The model under review builds one solid part; all positions refer to its coordinate system, in mm. A direction names the side the tool comes from. Coordinates: 2 decimals unless noted, no trailing zeros. Write each loop counter-clockwise with the first axis right and the second up, starting at its lowest first coordinate (ties: lowest second). Pieces come first, ordered by that corner, then holes.
```python
from build123d import *

# Parameters (mm, degrees)
SKETCH3_W = 6
SKETCH3_H = 2.2


with BuildPart() as part:
    # Sweep1: sweep along a path in Sketch1
    with BuildLine(Plane(origin=(0, 0, 0), x_dir=(0, 0, -1), z_dir=(1, 0, 0))) as sweep1_path:
        Line((0.31090006, -5.3474047), (403.879965212, 18.116247973))
        ThreePointArc((403.879965212, 18.116247973), (415.790396806, 31.112194288), (403.14572952, 43.394921614))
        Line((403.14572952, 43.394921614), (20.942535542, 43.394921614))
        ThreePointArc((20.942535542, 43.394921614), (13.956361094, 41.290814966), (9.294242947, 35.678457834))
        Line((9.294242947, 35.678457834), (-4.932278427, 2.089024985))
        ThreePointArc((-4.932278427, 2.089024985), (-4.377716999, -3.086582212), (0.31090006, -5.3474047))
    # Sketch3 → Sweep1 (sweep)
    with BuildSketch(Plane(origin=(0, 2.089024985, 4.932278427), x_dir=(1, 0, 0), z_dir=(0, -0.920813644, 0.390002863))):
        with Locations((0, 1.1)):
            Rectangle(SKETCH3_W, SKETCH3_H)
    sweep(path=sweep1_path.line)


solid = part.part
```
Item 1: Take a section at C-C, the plane z = -76.5. Write out the cut boundary in (x, y).
Solved:
outline: (-3, -3.12) - (3, -3.12) - (3, -0.92) - (-3, -0.92) - close; (-3, 43.39) - (3, 43.39) - (3, 45.59) - (-3, 45.59) - close
Item 2: To check wall thickness, follow line 1 along Y through (x, z) = (1.7, -47.5); line 2 along Y through (x, z) = (-2.2, -370); line 3 along Z through (x, y) = (-0.25, 30). State the ranges of each line that lie inside material, in increasing order.
Solved:
line 1: y = -4.81 to -2.6, 43.39 to 45.59
line 2: y = 13.94 to 16.15, 43.39 to 45.59
line 3: z = -417.98 to -415.77, -6.89 to -4.5
Item 3: Take a section at A-A, the plane y = 29. Write out the cut boundary in (x, z), plus the area to 3 significant figures.
Solved:
outline: (-3, -417.89) - (3, -417.89) - (3, -415.67) - (-3, -415.67) - close; (-3, -6.47) - (3, -6.47) - (3, -4.08) - (-3, -4.08) - close
area: 27.6 mm2
Item 4: Take a section at B-B, the plane x = -0.8. Write out the cut boundary in (y, z).
Solved:
outline: (-7.54, -0.44) - (15.92, -404.01) arc R14.85 ccw to (45.59, -403.15) - (45.59, -20.94) arc R14.85 ccw to (36.54, -7.27) - (2.95, 6.96) arc R7.56 ccw to start; hole (-5.35, -0.31) - (18.12, -403.88) arc R12.65 ccw to (43.39, -403.15) - (43.39, -20.94) arc R12.65 ccw to (35.68, -9.29) - (2.09, 4.93) arc R5.36 ccw to start
Item 5: Mouldability with a two-part tool opening along Z and no side actions: class faces 1 (the face through (-0.042, 30.856, -417.995)), 2 (the face through (0.042, 19.507, -0.056)), 3 (the face through (0.042, 30.839, -415.795)) as pulls with the +Z half, pulls with the -Z half, needs draft (parallel to the pull), parting line crosses it, or undercut.
Solved:
face 1: pulls with the -Z half
face 2: pulls with the +Z half
face 3: undercut
Item 6: Machinability: for faces 4 (the face through (0.042, 4.352, -205.048)), 5 (the face through (-0.04, 6.55, -204.92)), which of the approach directions +Z, -Z, +X, -X, +Y, -Y give a long, thin tool a straight path to every point of the face, cutting with its end or side? Answer none if there is none.
Solved:
face 4: -Z, +X, -X, -Y
face 5: +X, -X
Item 7: For pin 1 (1.5 mm diameter, centred on x = 0, y = 17.5, fed in from +Z); pin 2 (3 mm diameter, centred on x = 0.5, z = -181, fed in from -Y); pin 3 (3 mm diameter, centred on x = -2.5, z = -338, fed in from -Y), all flat-tipped, find the tip position at first contact; note any pin that passes through.
Solved:
pin 1: stops at z = 1.11
pin 2: stops at y = 2.87
pin 3: stops at y = 12
